from build123d import *

# Parameters (mm, degrees)
SKETCH_1_W      = 18
SKETCH_1_H      = 18
EXTRUDE_1_DEPTH = 50
EXTRUDE_2_DEPTH = 5


with BuildPart() as part:
    # 草图1 → 凸台-拉伸1 (new body)
    with BuildSketch(Plane(origin=(0, 0, 0), x_dir=(1, 0, 0), z_dir=(0, 1, 0))):
        Rectangle(SKETCH_1_W, SKETCH_1_H)
    extrude(amount=EXTRUDE_1_DEPTH)

    # 草图2 → 凸台-拉伸2 (add, symmetric)
    with BuildSketch(Plane(origin=(0, 0, 0), x_dir=(0, 0, -1), z_dir=(1, 0, 0))):
        with BuildLine():
            Line((-9, -10), (-9, 1.037830192))
            Line((-9, 1.037830192), (9, 1.037830192))
            Line((9, 1.037830192), (9, -10))
            ThreePointArc((9, -10), (0, -19), (-9, -10))
        make_face()
    extrude(amount=EXTRUDE_2_DEPTH, both=True)


solid = part.part
For this review, take the finished solid that the model builds, in its own axes (mm). A direction names the side the tool comes from. Round coordinates to 2 decimals unless told otherwise and drop trailing zeros. Write each loop counter-clockwise with the first axis right and the second up, starting at its lowest first coordinate (ties: lowest second). Pieces come first, ordered by that corner, then holes. Notation, with made-up numbers: (83.25, -29.75) -> (92.25, -29.75) arc R14 cw to (92.25, -8.75) -> close; hole circle Ø7 at (-10.5, -23). An arc over 180 degrees is marked (long way). Use CSV: the item, a comma, the result in double quotes.
(1) To check wall thickness, follow L1, parallel to Y at x = 6.75, z = 4.5; L2, parallel to X at y = -8, z = -1.75; L3, parallel to Y at x = -0.5, z = 7.5. State the ranges of each line that lie inside material, in increasing order. Write a range as [from, to].
Computed values:
L1,"[0, 50]"
L2,"[-5, 5]"
L3,"[-14.97, 50]"
(2) Clearance check with flat-ended pins moving along their axes: P1, Ø8, axis at x = 0, z = -4.5, coming from the -Y side; P2, Ø4.5, axis at x = 7.5, z = 3, coming from the -Y side; P3, Ø4.5, axis at x = -6, z = 3, coming from the -Y side. State where each tip first meets the part, or that it passes through.
Computed values:
P1,"y = -18.99"
P2,"y = 0"
P3,"y = -18.95"
(3) Consider section A-A, the plane z = 0. Give the boundary of the cut face in (x, y).
Computed values:
outline,"(-9, 0) -> (-5, 0) -> (-5, -19) -> (5, -19) -> (5, 0) -> (9, 0) -> (9, 50) -> (-9, 50) -> close"
(4) Consider section D-D, the plane z = -4.5. Give the boundary of the cut face in (x, y).
Computed values:
outline,"(-9, 0) -> (-5, 0) -> (-5, -17.79) -> (5, -17.79) -> (5, 0) -> (9, 0) -> (9, 50) -> (-9, 50) -> close"
(5) For faces 1 (the face through (5, -9, 0)), 2 (the face through (-5, -9, 0)), 3 (the face through (0, 20, -9)), list the 3-axis set-ups (+Z, -Z, +X, -X, +Y, -Y) from which the entire face can be reached by the end or side of a thin tool; tool diameter is ignored.
Computed values:
face 1,"+Z, -Z, +X, -Y"
face 2,"+Z, -Z, -X, -Y"
face 3,"-Z, +X, -X, +Y, -Y"
(6) Consider section B-B, the plane y = -4.5. Give the boundary of the cut face in (x, z), plus the area to 3 significant figures.
Computed values:
outline,"(-5, -9) -> (5, -9) -> (5, 9) -> (-5, 9) -> close"
area,"180 mm²"
(7) Consider section C-C, the plane x = -6.75. Give the boundary of the cut face in (y, z), plus the area to 3 significant figures.
Computed values:
outline,"(0, -9) -> (50, -9) -> (50, 9) -> (0, 9) -> close"
area,"900 mm²"
